from build123d import *

# Parameters (mm, degrees)
SKETCH_W        = 67
SKETCH_H        = 10
PAD_DEPTH       = 30
SKETCH001_W     = 37
SKETCH001_H     = 10
POCKET_DEPTH    = 20
FILLET_R        = 18.45
SKETCH002_R     = 3
POCKET001_DEPTH = 24
SKETCH003_R     = 1.9
POCKET002_DEPTH = 6


with BuildPart() as part:
    # Sketch → Pad (new body)
    with BuildSketch(Plane.XY):
        Rectangle(SKETCH_W, SKETCH_H)
    extrude(amount=PAD_DEPTH)

    # Sketch001 (on Face5 of Pad) → Pocket (cut)
    with BuildSketch(Plane(origin=(0, 0, 0), x_dir=(1, 0, 0), z_dir=(0, 0, -1))):
        Rectangle(SKETCH001_W, SKETCH001_H)
    extrude(amount=-POCKET_DEPTH, mode=Mode.SUBTRACT)

    # Fillet
    fillet_edges = [part.edges().sort_by_distance(p)[0] for p in [
        (-18.5, 0, 20),
        (18.5, 0, 20),
    ]]
    fillet(fillet_edges, radius=FILLET_R)

    # Sketch002 (on Face4 of Fillet) → Pocket001 (cut)
    with BuildSketch(Plane(origin=(0, 0, 0), x_dir=(1, 0, 0), z_dir=(0, 0, -1))):
        with Locations((-10, 0)):
            Circle(SKETCH002_R)
        with Locations((10, 0)):
            Circle(SKETCH002_R)
    extrude(amount=-POCKET001_DEPTH, mode=Mode.SUBTRACT)

    # Sketch003 (on Face8 of Pocket001) → Pocket002 (cut)
    with BuildSketch(Plane.XY.offset(30)):
        with Locations((-10, 0)):
            Circle(SKETCH003_R)
        with Locations((10, 0)):
            Circle(SKETCH003_R)
    extrude(amount=-POCKET002_DEPTH, mode=Mode.SUBTRACT)


solid = part.part
Design review of the part built by this model. Coordinates are the model's own, in mm. A direction names the side the tool comes from. Round coordinates to 2 decimals unless told otherwise and drop trailing zeros. Write each loop counter-clockwise with the first axis right and the second up, starting at its lowest first coordinate (ties: lowest second). Pieces come first, ordered by that corner, then holes. Notation, with made-up numbers: (77.25, 34.5) -> (122.25, 34.5) arc R20 cw to (122.25, 64.5) -> close; hole circle Ø8 at (5.25, -30). An arc over 180 degrees is marked (long way). One line per question, with ' | ' between items.
(1) Insertion check: P1, Ø3.5, axis at x = 10, y = 0, coming from the -Z side. The pin has a flat end and moves straight along its axis. Give the tip position at first contact, or say it passes through.
Result sheet:
P1: through
(2) Machinability: for faces 1 (the cylindrical face through (-13.24, -0.07, 14.45)), 2 (the flat face through (33.5, 0, 15)), 3 (the flat face through (12, 1, 24)), which of the approach directions +Z, -Z, +X, -X, +Y, -Y give a long, thin tool a straight path to every point of the face, cutting with its end or side? Answer none if there is none.
Result sheet:
face 1: -Z, +Y, -Y | face 2: +Z, -Z, +X, +Y, -Y | face 3: -Z
(3) Take a section at C-C, the plane z = 9.25. State the section outline as (x, y) points, and give its area (3 significant figures).
Result sheet:
outline: (-33.5, -5) -> (-16.82, -5) -> (-16.82, 5) -> (-33.5, 5) -> close; (16.82, -5) -> (33.5, -5) -> (33.5, 5) -> (16.82, 5) -> close | area: 334 mm2
(4) Take a section at B-B, the plane y = 1. State the section outline as (x, z) points.
Result sheet:
outline: (-33.5, 0) -> (-18.5, 0) -> (-18.5, 1.55) arc R18.45 cw to (-12.83, 14.86) -> (-12.83, 24) -> (-11.62, 24) -> (-11.62, 30) -> (-33.5, 30) -> close; (-8.38, 24) -> (-7.17, 24) -> (-7.17, 18.57) arc R18.45 cw to (-0.05, 20) -> (0.05, 20) arc R18.45 cw to (7.17, 18.57) -> (7.17, 24) -> (8.38, 24) -> (8.38, 30) -> (-8.38, 30) -> close; (11.62, 24) -> (12.83, 24) -> (12.83, 14.86) arc R18.45 cw to (18.5, 1.55) -> (18.5, 0) -> (33.5, 0) -> (33.5, 30) -> (11.62, 30) -> close
(5) Take a section at A-A, the plane x = -10. State the section outline as (y, z) points, and give its area (3 significant figures).
Result sheet:
outline: (-5, 17.09) -> (-3, 17.09) -> (-3, 24) -> (-1.9, 24) -> (-1.9, 30) -> (-5, 30) -> close; (1.9, 24) -> (3, 24) -> (3, 17.09) -> (5, 17.09) -> (5, 30) -> (1.9, 30) -> close | area: 64.9 mm2
(6) Draft analysis for pull direction Y (two halves, no side actions). For faces 4 (the flat face through (0, 5, 21)), 5 (the cylindrical face through (11.755, -0.728, 27.042)), 6 (the flat face through (18.5, 0, 1)), state which applies: released by +Y, released by -Y, zero draft, split by the parting line, or undercut.
Result sheet:
face 4: released by +Y | face 5: undercut | face 6: zero draft
(7) Wall thickness on line 1 (X direction, y = 0, z = 17.5); line 2 (Y direction, x = 10, z = 19.5); line 3 (Y direction, x = 10, z = 26.85): over which ranges is each line inside the solid? List them lowest first. Write a range as [from, to].
Result sheet:
line 1: [-33.5, -13], [13, 33.5] | line 2: [-5, -3], [3, 5] | line 3: [-5, -1.9], [1.9, 5]
(8) Take a section at D-D, the plane z = 22.75. State the section outline as (x, y) points.
Result sheet:
outline: (-33.5, -5) -> (33.5, -5) -> (33.5, 5) -> (-33.5, 5) -> close; hole circle Ø6 at (-10, 0); hole circle Ø6 at (10, 0)
